from build123d import *

# Parameters (mm, degrees)
SKETCH1_R                                    = 17
SKETCH1_R_2                                  = 8
BOSS_EXTRUDE4_DEPTH                          = 2
REVOLVE2_ANGLE                               = 40
CIRPATTERN1_COUNT                            = 3
FILLET1_R                                    = 5
CSK_FOR_M2_COUNTERSUNK_FLAT_HEAD_SCR_2_COUNT = 2
CSK_FOR_M2_COUNTERSUNK_FLAT_HEAD_SCR_2_PITCH = 20.784609691
CSK_FOR_M2_COUNTERSUNK_FLAT_HEAD_SCR_3_COUNT = 2
CSK_FOR_M2_COUNTERSUNK_FLAT_HEAD_SCR_3_PITCH = 20.747553677
BOSS_EXTRUDE6_DEPTH                          = 14


with BuildPart() as part:
    # Sketch1 → Boss-Extrude4 (new body)
    with BuildSketch(Plane(origin=(0, 0, 0), x_dir=(1, 0, 0), z_dir=(0, 1, 0))):
        with Locations(Location((0, 0, 0), (0, 0, 270))):
            Circle(SKETCH1_R)
        with Locations(Location((0, 0, 0), (0, 0, 270))):
            Circle(SKETCH1_R_2, mode=Mode.SUBTRACT)
    extrude(amount=BOSS_EXTRUDE4_DEPTH)

    # Sketch5 → Revolve2 (revolve)
    with BuildSketch(Plane.XY):
        Polygon((-17, 0), (-22, 0), (-21, 15), (-17, 15), align=None)
    revolve2 = revolve(axis=Axis((0, 9.813682869, 0), (0, -1, 0)), revolution_arc=REVOLVE2_ANGLE)

    # CirPattern1: Revolve2 ×3 about axis
    cirpattern1_axis = Axis((0, 0, 0), (0, 1, 0))
    for i in range(1, CIRPATTERN1_COUNT):
        add(revolve2.rotate(cirpattern1_axis, i * 360 / CIRPATTERN1_COUNT))

    # Fillet1
    fillet1_edges = [part.edges().sort_by_distance(p)[0] for p in [
        (-13.022755533, 1, -10.927389365),
        (-17, 1, 0),
        (-2.95201902, 1, 16.741731801),
        (8.5, 1, 14.722431864),
        (15.974774553, 1, -5.814342437),
        (8.5, 1, -14.722431864),
    ]]
    fillet(fillet1_edges, radius=FILLET1_R)

    # Sketch13 → CSK for M2 Countersunk Flat Head Screw1 (revolve, cut)
    with BuildSketch(Plane(origin=(2.083778132, 2, 11.817693036), x_dir=(0, 0, 1), z_dir=(1, 0, 0))):
        Polygon((0, 0), (0, 2), (1.2, 2), (1.2, 1), (2.2, 0), align=None)
    csk_for_m2_countersunk_flat_head_screw1 = revolve(axis=Axis((2.083778132, 8.35, 11.817693036), (0, -1, 0)), mode=Mode.SUBTRACT)

    # CSK for M2 Countersunk Flat Head Scr 2: CSK for M2 Countersunk Flat Head Screw1 ×2
    with Locations(*[Vector(0.3420201433256633, 0, -0.9396926207859104) * (i * CSK_FOR_M2_COUNTERSUNK_FLAT_HEAD_SCR_2_PITCH) for i in range(1, CSK_FOR_M2_COUNTERSUNK_FLAT_HEAD_SCR_2_COUNT)]):
        add(csk_for_m2_countersunk_flat_head_screw1, mode=Mode.SUBTRACT)

    # CSK for M2 Countersunk Flat Head Scr 3: CSK for M2 Countersunk Flat Head Screw1 ×2
    with Locations(*[Vector(-0.6419971087705412, 0, -0.7667070577021357) * (i * CSK_FOR_M2_COUNTERSUNK_FLAT_HEAD_SCR_3_PITCH) for i in range(1, CSK_FOR_M2_COUNTERSUNK_FLAT_HEAD_SCR_3_COUNT)]):
        add(csk_for_m2_countersunk_flat_head_screw1, mode=Mode.SUBTRACT)

    # Sketch24 → Boss-Extrude6 (add)
    with BuildSketch(Plane(origin=(0, 2, 0), x_dir=(1, 0, 0), z_dir=(0, 1, 0))):
        with BuildLine():
            ThreePointArc((12.528097784, 11.491160338), (12.448209945, 10.445288373), (13.492065142, 10.342348776))
            ThreePointArc((13.492065142, 10.342348776), (13.022755533, 10.927389365), (12.528097784, 11.491160338))
        make_face()
    extrude(amount=BOSS_EXTRUDE6_DEPTH)


solid = part.part
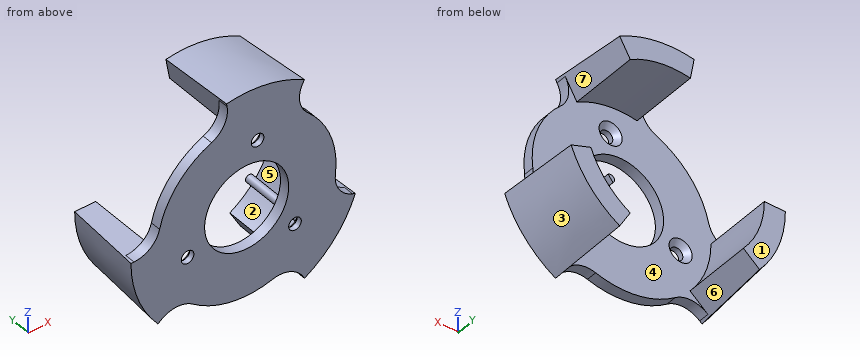
Here's how the part is built. I have some questions about the finished solid (model axes, mm). Face numbers are marked on the shaded views. A direction names the side the tool comes from. Round coordinates to 2 decimals unless told otherwise and drop trailing zeros. Loops run counter-clockwise (first coordinate to the right, second up) from the corner with the lowest first, then second, coordinate; pieces in that order, holes last. Notation, with made-up numbers: (-31, 76) - (-15, 76) arc R24 cw to (-15, 87) - close; hole circle Ø6 at (-39.5, 36). An arc over 180 degrees is marked (long way). One line per question, with ' | ' between items. Start each with the question number.
Q1. I want a section at A-A (y = 10.5). Write out the boundary of the cut face in (x, z), then the cut area to 3 significant figures.
Q2. Please list where these lines run through material, in increasing order: line 1 (Y direction, x = 17, z = -4); line 2 (Z direction, x = -1.5, y = 1); line 3 (X direction, y = 1, z = 1). Write a range as [from, to].
Q3. I want a section at B-B (z = 2.5). Write out the boundary of the cut face in (x, y), then the cut area to 3 significant figures.
Q4. We'd pull the mould along Z, two halves only. Please class the marked faces 1, 2 and 3: +Z half, -Z half, draft (parallel to the pull), parting line (faces both ways), or undercut.
Q5. For the marked faces 4, 5, 6 and 7, which set-ups out of +Z, -Z, +X, -X, +Y, -Y let a thin tool reach every point of the face, with its end or its side?
Q6. I want a section at C-C (y = 3.25). Write out the boundary of the cut face in (x, z), then the cut area to 3 significant figures.
Q7. Will these pins go through, and if not, where does the flat tip stop? pin 1 (13 mm diameter, centred on x = 0, z = 0, fed in from -Y); pin 2 (4 mm diameter, centred on x = 9.19, z = -7.71, fed in from +Y); pin 3 (7 mm diameter, centred on x = 2, z = 18.5, fed in from +Y); pin 4 (2 mm diameter, centred on x = 9, y = 4, fed in from -Z).
Response values:
1) outline: (-21.3, 0) arc R21.3 ccw to (-16.32, -13.69) - (-13.02, -10.93) arc R17 cw to (-17, 0) - close; (-3.7, 20.98) - (-2.95, 16.74) arc R17 cw to (8.5, 14.72) - (10.65, 18.45) arc R21.3 ccw to start; (8.5, -14.72) - (10.65, -18.45) arc R21.3 ccw to (20.02, -7.29) - (15.97, -5.81) arc R17 cw to (13.49, -10.34) arc R0.75 ccw to (12.53, -11.49) arc R17 cw to start | area: 173 mm²
2) line 1: y = [0, 2] | line 2: z = [-16.93, -7.86], [7.86, 21.88] | line 3: x = [-18.42, -7.94], [7.94, 16.97]
3) outline: (-17.09, 0) - (-7.6, 0) - (-7.6, 2) - (-17.09, 2) - close; (7.6, 0) - (16.82, 0) - (16.82, 2) - (7.6, 2) - close | area: 37.4 mm²
4) face 1: draft | face 2: undercut | face 3: -Z half
5) face 4: +Y | face 5: +Z, +Y | face 6: -Z, +Y | face 7: +X, +Y
6) outline: (-21.78, 0) arc R21.78 ccw to (-16.69, -14) - (-13.02, -10.93) arc R17 cw to (-17, 0) - close; (-3.78, 21.45) - (-2.95, 16.74) arc R17 cw to (8.5, 14.72) - (10.89, 18.86) arc R21.78 ccw to start; (8.5, -14.72) - (10.89, -18.86) arc R21.78 ccw to (20.47, -7.45) - (15.97, -5.81) arc R17 cw to (13.49, -10.34) arc R0.75 ccw to (12.53, -11.49) arc R17 cw to start | area: 195 mm²
7) pin 1: passes through | pin 2: stops at y = 1.8 | pin 3: stops at y = 15 | pin 4: stops at z = -17.32
